Model file for the job. Use its own axes, mm. A direction names the side the tool comes from. Give positions to 0.01 mm unless a question says otherwise; leave off trailing zeros. Write each loop counter-clockwise with the first axis right and the second up, starting at its lowest first coordinate (ties: lowest second). Pieces come first, ordered by that corner, then holes.
```python
from build123d import *

# Parameters (mm, degrees)
SKETCH1_R           = 1.96
BOSS_EXTRUDE1_DEPTH = 10
SKETCH2_R           = 3.55
BOSS_EXTRUDE2_DEPTH = 4
CUT_EXTRUDE1_DEPTH  = 2


with BuildPart() as part:
    # Sketch1 → Boss-Extrude1 (new body)
    with BuildSketch(Plane.XY):
        Circle(SKETCH1_R)
    extrude(amount=BOSS_EXTRUDE1_DEPTH)

    # Sketch2 → Boss-Extrude2 (add)
    with BuildSketch(Plane.XY.offset(10)):
        Circle(SKETCH2_R)
    extrude(amount=BOSS_EXTRUDE2_DEPTH)

    # Sketch3 → Cut-Extrude1 (cut)
    with BuildSketch(Plane.XY.offset(14)):
        Polygon((1.325823406, 1.114536808), (-0.302305486, 1.705465155), (-1.628128892, 0.590928347), (-1.325823406, -1.114536808), (0.302305486, -1.705465155), (1.628128892, -0.590928347), align=None)
    extrude(amount=-CUT_EXTRUDE1_DEPTH, mode=Mode.SUBTRACT)


solid = part.part
```
1. Which spindle directions (+Z, -Z, +X, -X, +Y, -Y) get a long thin tool onto all of the face, cutting with end or side? Do faces 4 (the flat face through (-0.523, -1.406, 13.014)), 5 (the flat face through (2, -2, 10)), 6 (the cylindrical face through (-0.46, 3.52, 11.97)). Say none if no direction does.
Calculated:
face 4: +Z
face 5: -Z
face 6: +Z, -Z
2. Slice it at C-C, the plane y = 0. Write the cut outline in (x, z), and give its area (3 significant figures).
Calculated:
outline: (-3.55, 10) - (-1.96, 10) - (-1.96, 0) - (1.96, 0) - (1.96, 10) - (3.55, 10) - (3.55, 14) - (1.52, 14) - (1.52, 12) - (-1.52, 12) - (-1.52, 14) - (-3.55, 14) - close
area: 61.5 mm2
3. Slice it at D-D, the plane z = 5. Write the cut outline in (x, y).
Calculated:
outline: circle Ø3.92 at (0, 0)
4. Slice it at A-A, the plane z = 12.5. Write the cut outline in (x, y), and give its area (3 significant figures).
Calculated:
outline: circle Ø7.1 at (0, 0); hole (-1.63, 0.59) - (-1.33, -1.11) - (0.3, -1.71) - (1.63, -0.59) - (1.33, 1.11) - (-0.3, 1.71) - close
area: 31.8 mm2
5. Probe probe 1 along Z at (x, y) = (-0.5, -1); probe 2 along Y at (x, z) = (-0.5, 12.5); probe 3 along Z at (x, y) = (0.75, -2.25). List the from-to ranges inside material, lowest first.
Calculated:
probe 1: z = 0 to 12
probe 2: y = -3.51 to -1.41, 1.54 to 3.51
probe 3: z = 10 to 14
6. Slice it at B-B, the plane x = 1. Write the cut outline in (y, z).
Calculated:
outline: (-3.41, 10) - (-1.69, 10) - (-1.69, 0) - (1.69, 0) - (1.69, 10) - (3.41, 10) - (3.41, 14) - (1.23, 14) - (1.23, 12) - (-1.12, 12) - (-1.12, 14) - (-3.41, 14) - close
7. Pull direction Y, two halves, no side cores. Call faces 1 (the flat face through (2, 0, 14)), 2 (the cylindrical face through (-0.425, -1.913, 4.93)), 3 (the flat face through (0.523, 1.406, 13.014)): +Y half, -Y half, draft (parallel to the pull), parting line (faces both ways), or undercut.
Calculated:
face 1: draft
face 2: parting line
face 3: undercut
8. Pin check, flat tips, straight feed: P1, Ø4, axis at x = 2.5, z = 9, coming from the +Y side; P2, Ø1, axis at y = -2, z = 4, coming from the -X side; P3, Ø3, axis at x = 1.5, z = 3.5, coming from the -Y side. Stop position of each tip, or through.
Calculated:
P1: stops at y = 3.47
P2: stops at x = -1.26
P3: stops at y = -1.96
